Here's how the part is built. I have some questions about the finished solid (model axes, mm). A direction names the side the tool comes from. Give positions to 0.01 mm unless a question says otherwise; leave off trailing zeros. Write each loop counter-clockwise with the first axis right and the second up, starting at its lowest first coordinate (ties: lowest second). Pieces come first, ordered by that corner, then holes. Notation, with made-up numbers: M -26.5,-22 L 9.5,-22 A14 ccw 9.5,-18 Z; hole C -4,22 d9. An arc over 180 degrees is marked long. Answer as CSV lines item,"result". Start each with the question number.
Q1. Suppose I cut it at C-C (x = -57). Write out the boundary of the cut face in (y, z), then the cut area to 3 significant figures.
Q2. Thinking about a two-plate mould opening in Z: for faces 1 (the conical face through (-68.213, 0.201, -9.083)), 2 (the flat face through (-84.79, 1, -3)), 3 (the cylindrical face through (-91.72, 4.65, 1.03)), which applies, +Z half, -Z half, draft (parallel to the pull), parting line (faces both ways), or undercut?
Q3. For pin 1 (2 mm diameter, centred on y = 0, z = 9, fed in from -X); pin 2 (8 mm diameter, centred on x = -22.5, y = -1.5, fed in from +Z); pin 3 (12 mm diameter, centred on x = -21, z = -7, fed in from -Y), each with a flat end and sliding along its axis, tell me the tip position at first contact or that it passes through.
Q4. If I drill on line 1 along Y through (x, z) = (-75.75, 0); line 2 along X through (y, z) = (3.25, -1.5); line 3 along X through (y, z) = (-5, -7.5), over which ranges is the centre line in solid material (lowest first)?
Q5. On a 3-axis mill with a long thin cutter (end or side, diameter ignored), from which of +Z, -Z, +X, -X, +Y, -Y can I reach the whole of each face in a straight line? I mean faces 4 (the cylindrical face through (-75.27, -0.16, -7.76)), 5 (the flat face through (-95.584, 0, 0)), 6 (the cylindrical face through (-36.24, -3.01, -9.55)). Say none if no direction works.
Q6. Suppose I cut it at B-B (x = -83). Write out the boundary of the cut face in (y, z).
Q7. Suppose I cut it at A-A (x = -72). Write out the boundary of the cut face in (y, z).
```python
from build123d import *

# Parameters (mm, degrees)
CIRPATTERN1_COUNT = 4


with BuildPart() as part:
    # Sketch1 → Revolve1 (revolve)
    with BuildSketch(Plane.XY, mode=Mode.PRIVATE) as revolve1_sk:
        Polygon((-95.584028604, 0), (-95.584028604, 4.7625), (-87.964028604, 4.7625), (-87.964028604, 2.9972), (-84.790088556, 2.9972), (-84.790088556, 6.0071), (-81.534, 6.0071), (-81.534, 10.9855), (-60.269072576, 10.9855), (-60.269072576, 10.013003393), (-12.869596711, 10.013003393), (-12.869596711, 10.9855), (0, 10.9855), (0, 0), align=None)
    revolve(revolve1_sk.sketch.rotate(Axis((0, 0, 0), (-1, 0, 0)), 90), axis=Axis((0, 0, 0), (-1, 0, 0)))

    # Sketch3 → M3x0.5 Tapped Hole1 (revolve, cut)
    with BuildSketch(Plane(origin=(-81.534, 9, 0), x_dir=(0, 0, 1), z_dir=(0, 1, 0))):
        Polygon((0, 0), (0, 13.451075774), (1.25, 12.7), (1.25, 0), align=None)
    m3x0_5_tapped_hole1 = revolve(axis=Axis((-87.884, 9, 0), (1, 0, 0)), mode=Mode.SUBTRACT)

    # CirPattern1: M3x0.5 Tapped Hole1 ×4 about axis
    cirpattern1_axis = Axis((0, 0, 0), (1, 0, 0))
    for i in range(1, CIRPATTERN1_COUNT):
        add(m3x0_5_tapped_hole1.rotate(cirpattern1_axis, i * 360 / CIRPATTERN1_COUNT), mode=Mode.SUBTRACT)


solid = part.part
```
Resolved:
1,outline,"C 0,0 d20.03"
1,area,"315 mm^2"
2,face 1,"undercut"
2,face 2,"draft"
2,face 3,"parting line"
3,pin 1,"x = -68.68"
3,pin 2,"z = 10.01"
3,pin 3,"y = -9.96"
4,line 1,"-10.99 to -10.25, -7.75 to 7.75, 10.25 to 10.99"
4,line 2,"-95.58 to -87.96, -84.79 to 0"
4,line 3,"-81.53 to 0"
5,face 4,"-X"
5,face 5,"+Z, -Z, -X, +Y, -Y"
5,face 6,"none"
6,outline,"C 0,0 d12.01"
7,outline,"C 0,0 d21.97; hole C -9,0 d2.5; hole C 0,-9 d2.5; hole C 0,9 d2.5; hole C 9,0 d2.5"
